from build123d import *

# Parameters (mm, degrees)
BASE_DEPTH      = 1
SKETCH_2_W      = 5
SKETCH_2_H      = 4.241016002
SKETCH_2_W_2    = 3.399648754
SKETCH_2_H_2    = 3.069015748
SKETCH_2_W_3    = 8.833032766
SKETCH_2_H_3    = 2.239343378
SKETCH_2_W_4    = 7
SKETCH_2_H_4    = 1.440284481
SKETCH_2_W_5    = 2.346977394
SKETCH_2_H_5    = 6.402667005
SKETCH_2_W_6    = 4.921188948
SKETCH_2_H_6    = 7.755318771
SKETCH_2_W_7    = 1.992801626
SKETCH_2_H_7    = 3.770694824
PILLARS_DEPTH   = 2.2
SKETCH_3_W      = 1.5
SKETCH_3_H      = 8
SKETCH_3_W_2    = 29.4
SKETCH_3_H_2    = 1.268554838
SKETCH_3_W_3    = 6.4
SKETCH_3_H_3    = 1.412663195
ENCLOSURE_DEPTH = 3.800051
PADDING_REACH   = 5.2
SKETCH_5_W      = 1.992801626
SKETCH_5_H      = 0.414508298
SKETCH_5_W_2    = 4.921188948
SKETCH_5_H_2    = 0.244108357
SKETCH_5_W_3    = 0.1
SKETCH_5_H_3    = 4.241016002


with BuildPart() as part:
    # 草图1 → Base (new body)
    with BuildSketch(Plane.XY):
        Polygon((14.65, 20), (-14.65, 20), (-17.65, 17), (-17.65, -17), (-14.65, -20), (-8.35, -20), (-8.35, -14), (17.65, -14), (17.65, 6.919667259), (12.305816612, 6.919667259), (12.305816612, 16.420619761), (17.65, 16.420619761), (17.65, 17), align=None)
    extrude(amount=BASE_DEPTH)

    # 草图2 → Pillars (add)
    with BuildSketch(Plane.XY.offset(1)):
        with Locations((-12.199329439, -5.609511049)):
            Rectangle(SKETCH_2_W, SKETCH_2_H)
        with Locations((-8.825830005, 3.993507112)):
            Rectangle(SKETCH_2_W_2, SKETCH_2_H_2)
        with Locations((3.599511049, -3.092672705)):
            Rectangle(SKETCH_2_W_3, SKETCH_2_H_3)
        with Locations((3.303022606, 1.942635256)):
            Rectangle(SKETCH_2_W_4, SKETCH_2_H_4)
        with Locations((16.476511303, 3.718333757)):
            Rectangle(SKETCH_2_W_5, SKETCH_2_H_5)
        with Locations((9.845222138, 14.60967742)):
            Rectangle(SKETCH_2_W_6, SKETCH_2_H_6)
        with Locations((-13.702928626, 16.431589452)):
            Rectangle(SKETCH_2_W_7, SKETCH_2_H_7)
    extrude(amount=PILLARS_DEPTH)

    # 草图3 → Enclosure (add)
    with BuildSketch(Plane.XY.offset(1)):
        with Locations((-15.549329439, 10)):
            Rectangle(SKETCH_3_W, SKETCH_3_H)
        with Locations((0, 19.365722581)):
            Rectangle(SKETCH_3_W_2, SKETCH_3_H_2)
        with Locations((-11.5, -19.293668402)):
            Rectangle(SKETCH_3_W_3, SKETCH_3_H_3)
        with Locations((-15.549329439, -6)):
            Rectangle(SKETCH_3_W, SKETCH_3_H)
    extrude(amount=ENCLOSURE_DEPTH)

    # 草图5 → Padding (add, up to next)
    with BuildSketch(Plane.XY.offset(3.2), mode=Mode.PRIVATE) as padding_sk1:
        with Locations((-13.702928626, 18.524191013)):
            Rectangle(SKETCH_5_W, SKETCH_5_H)
    padding_tool1 = extrude(padding_sk1.sketch, amount=-PADDING_REACH, mode=Mode.PRIVATE) - part.part
    add(padding_tool1.solids().sort_by_distance((-13.702929, 18.524191, 3.2))[0])
    # 草图5 → Padding (add, up to next)
    with BuildSketch(Plane.XY.offset(3.2), mode=Mode.PRIVATE) as padding_sk2:
        with Locations((9.845222138, 18.609390983)):
            Rectangle(SKETCH_5_W_2, SKETCH_5_H_2)
    padding_tool2 = extrude(padding_sk2.sketch, amount=-PADDING_REACH, mode=Mode.PRIVATE) - part.part
    add(padding_tool2.solids().sort_by_distance((9.845222, 18.609391, 3.2))[0])
    # 草图5 → Padding (add, up to next)
    with BuildSketch(Plane.XY.offset(3.2), mode=Mode.PRIVATE) as padding_sk3:
        with Locations((-14.749329439, -5.609511049)):
            Rectangle(SKETCH_5_W_3, SKETCH_5_H_3)
    padding_tool3 = extrude(padding_sk3.sketch, amount=-PADDING_REACH, mode=Mode.PRIVATE) - part.part
    add(padding_tool3.solids().sort_by_distance((-14.749329, -5.609511, 3.2))[0])


solid = part.part
Build history of the part. All positions in model axes, mm. A direction names the side the tool comes from. Round coordinates to 2 decimals unless told otherwise and drop trailing zeros. Write each loop counter-clockwise with the first axis right and the second up, starting at its lowest first coordinate (ties: lowest second). Pieces come first, ordered by that corner, then holes. Notation, with made-up numbers: M -11,-12.75 L 47,-12.75 A20 ccw 47,-2.75 Z; hole C 38,21.25 d11. An arc over 180 degrees is marked long. Answer as a JSON object with one key per item and string values. Group by question number.
(1) Mould opens along X. For faces 1 (the flat face through (16.17, 18.48, 0.49)), 2 (the flat face through (-14.799, 10, 3)), 3 (the flat face through (3, 2, 3.2)), 4 (the flat face through (-10.526, 4, 2)) say: pulls with the +X half, pulls with the -X half, needs draft (parallel to the pull), parting line crosses it, or undercut.
(2) Cut at A-A (x = 2.5). Give the cut face in (y, z).
(3) Flat gauge pins, fed straight in: pin 1 (0.7 mm diameter, centred on x = -16, z = 2.5, fed in from +Y); pin 2 (1.1 mm diameter, centred on y = 8.5, z = 2, fed in from +X); pin 3 (1 mm diameter, centred on x = -13.5, y = 17.5, fed in from +Z). Where does each tip first touch, or does it go through?
(4) Drill centre lines: L1, parallel to Y at x = 0, z = 2.8; L2, parallel to X at y = 15.5, z = 2.1; L3, parallel to Y at x = 6.5, z = 3.5. Where is each one in solid material? Low to high.
(5) Cut at C-C (y = -8.5). Give the cut face in (x, z), and give its area (3 significant figures).
(6) Which spindle directions (+Z, -Z, +X, -X, +Y, -Y) get a long thin tool onto all of the face, cutting with end or side? Do faces 5 (the flat face through (16, 0.517, 2)), 6 (the flat face through (-16, 14, 3)), 7 (the flat face through (-0.817, -3, 2)). Say none if no direction does.
(7) Cut at B-B (z = 4.3). Give the cut face in (x, y).
(8) Cut at D-D (z = 1.85). Give the number of separate pieces and of enclosed holes in the cut face, and give its area (3 significant figures).
Responses:
{
 "1": {"face 1": "pulls with the +X half", "face 2": "undercut", "face 3": "needs draft", "face 4": "pulls with the -X half"},
 "2": {"outline": "M -14,0 L 20,0 L 20,4.8 L 18.73,4.8 L 18.73,1 L 2.66,1 L 2.66,3.2 L 1.22,3.2 L 1.22,1 L -1.97,1 L -1.97,3.2 L -4.21,3.2 L -4.21,1 L -14,1 Z"},
 "3": {"pin 1": "stops at y = 14", "pin 2": "stops at x = -14.8", "pin 3": "stops at z = 3.2"},
 "4": {"L1": "y = -4.21 to -1.97, 1.22 to 2.66, 18.73 to 20", "L2": "x = -14.7 to -12.71, 7.38 to 12.31", "L3": "y = 18.73 to 20"},
 "5": {"outline": "M -17.65,0 L 17.65,0 L 17.65,1 L -14.8,1 L -14.8,4.8 L -16.3,4.8 L -16.3,1 L -17.65,1 Z", "area": "41.0 mm2"},
 "6": {"face 5": "+Z, +X, -X, -Y", "face 6": "+Z, -X, +Y", "face 7": "+Z, -Y"},
 "7": {"outline": "M -16.3,-10 L -14.8,-10 L -14.8,-2 L -16.3,-2 Z; M -16.3,6 L -14.8,6 L -14.8,14 L -16.3,14 Z; M -14.7,-20 L -8.3,-20 L -8.3,-18.59 L -14.7,-18.59 Z; M -14.7,18.73 L 14.7,18.73 L 14.7,20 L -14.7,20 Z"},
 "8": {"separate pieces": "8", "enclosed holes": "0", "area": "195 mm2"}
}
